Autodesk Inventor part; units mm, degrees
ref_plane "YZ Plane" through (0, 0, 0) normal (1, 0, 0) x (0, 1, 0)
ref_plane "XZ Plane" through (0, 0, 0) normal (0, 1, 0) x (-1, 0, 0)
ref_plane "XY Plane" through (0, 0, 0) normal (0, 0, 1) x (1, 0, 0)
sketch "スケッチ1" plane through (0, 0, 0) normal (0, 0, 1) x (1, 0, 0)
  line L0 (-157.5, 1000) -> (-142.5, 1000)
  line L1 (-142.5, 1000) -> (-142.5, 0)
  line L2 (-142.5, 0) -> (-157.5, 0)
  line L3 (-157.5, 0) -> (-157.5, 1000)
  line L4 (142.5, 500) -> (157.5, 500) construction
  line L5 (157.5, 500) -> (157.5, 0) construction
  line L6 (157.5, 0) -> (142.5, 0)
  line L7 (142.5, 0) -> (142.5, 500) construction
  circle A0 centre (-150, 0) radius 1.6
  circle A1 centre (150, 500) radius 1.6
  line L8 (127.3377, 476.8069) -> (140.2001, 469.0894) construction
  line L9 (140.2001, 469.0894) -> (-127.3377, 23.1931) construction
  line L10 (-127.3377, 23.1931) -> (-140.2001, 30.9106)
  line L11 (-140.2001, 30.9106) -> (127.3377, 476.8069) construction
  line L12 (-150, 0) -> (-133.7689, 27.0518) construction
  circle A2 centre (-150, 1000) radius 1.6
  circle A3 centre (150, 490) radius 1.6
  line L13 (133.7689, 472.9482) -> (150, 500) construction
  line L14 (-133.7689, 27.0518) -> (133.7689, 472.9482) construction
  circle A4 centre (128.6239, 464.3732) radius 1.6
  circle A5 centre (123.479, 455.7983) radius 1.6
  circle A6 centre (118.334, 447.2234) radius 1.6
  circle A7 centre (150, 510) radius 1.6
  circle A8 centre (128.6239, 535.6268) radius 1.6
  circle A9 centre (123.479, 544.2017) radius 1.6
  circle A10 centre (118.334, 552.7766) radius 1.6
  line L15 (157.5, 517.5) -> (157.5, 482.5)
  line L16 (157.5, 482.5) -> (148.2464, 482.5)
  line L17 (157.5, 517.5) -> (148.2464, 517.5)
  line L18 (148.2464, 517.5) -> (120.9065, 563.0665)
  line L19 (120.9065, 563.0665) -> (108.0441, 555.3491)
  line L20 (108.0441, 555.3491) -> (136.6231, 507.7174)
  line L21 (148.2464, 482.5) -> (120.9065, 436.9335)
  line L22 (120.9065, 436.9335) -> (108.0441, 444.6509)
  line L23 (108.0441, 444.6509) -> (136.6231, 492.2826)
  arc A11 (136.6231, 492.2826) -> (136.6231, 507.7174) centre (123.7607, 500) ccw
  line L24 (118.334, 552.7766) -> (128.6239, 535.6268) construction
  point P0 (0, 0)
  point P1 (150, 0)
  dimension "d0" = 15
  dimension "d1" = 15
  dimension "d2" = 1000
  dimension "d3" = 500
  dimension "d4" = 3.2
  dimension "d5" = 3.2
  dimension "d6" = 285
  dimension "d7" = 142.5
  dimension "d8" = 15
  dimension "d9" = 7.5
  dimension "d10" = 520
  dimension "d11" = 3.2
  dimension "d12" = 3.2
  dimension "d13" = 10
  dimension "d14" = 3.2
  dimension "d15" = 3.2
  dimension "d16" = 3.2
  dimension "d17" = 10
  dimension "d18" = 10
  dimension "d19" = 10
  dimension "d20" = 3.2
  dimension "d21" = 10
  dimension "d22" = 7.5
  dimension "d23" = 7.5
  dimension "d24" = 7.5
  dimension "d25" = 7.5
  dimension "d26" = 7.5
  dimension "d27" = 7.5
  dimension "d28" = 7.5
  dimension "d30" = 7.5
  dimension "d31" = 7.5
  dimension "d32" = 15
extrude "押し出し1" add sketch "スケッチ1" along normal blind 3 contours L15 L16 L21 L22 L23 A11 L20 L19 L18 L17
fillet "フィレット1" radius 2 8 edges at (120.9065, 563.0665, 1.5) (157.5, 517.5, 1.5) (157.5, 482.5, 1.5) (120.9065, 436.9335, 1.5) (108.0441, 444.6509, 1.5) (148.2464, 482.5, 1.5) (148.2464, 517.5, 1.5) (108.0441, 555.3491, 1.5)
properties part number "プレート保持_固定具2" material "アルミニウム 6061"
Part model, mm, in its own coordinate system. A direction names the side the tool comes from. Round coordinates to 2 decimals unless told otherwise and drop trailing zeros. Order: outer loops, then holes, each group sorted by start corner. A loop starts at its lowest first (then second) coordinate and runs counter-clockwise, first axis right, second up. Notation, with made-up numbers: M 88,-14.5 L 105,-14.5 A24 ccw 105,21.5 Z; hole C 40.25,-36.75 d9. An arc over 180 degrees is marked long. Put each result on its own line as item: value. Start each with the question number.
1. Drill centre lines: probe 1 along Y at (x, z) = (150, 1.1); probe 2 along Y at (x, z) = (119, 2.7); probe 3 along X at (y, z) = (500, 0.75). Where is each one in solid material? Low to high. Write a range as [from, to].
2. Slice it at A-A on y = 500. List the corners of the cut face in (x, z).
3. Slice it at B-B on z = 2.1. State how many separate pieces and enclosed holes the cut face has, then the cut area to 3 significant figures.
4. Two-plate mould, pull along X, no slides. Class faces 4 (the face through (122.655, 530.997, 1.479)), 5 (the face through (120.68, 437.73, 1.52)), 6 (the face through (128.416, 462.787, 1.479)): +X half, -X half, draft (parallel to the pull), parting line (faces both ways), or undercut.
5. Slice it at C-C on x = 114.5. List the corners of the cut face in (y, z).
6. Tool access for faces 1 (the face through (114.541, 440.753, 1.479)), 2 (the face through (152, 482.5, 1)), 3 (the face through (122.655, 469.003, 1.479)): list every direction of +Z, -Z, +X, -X, +Y, -Y with a clear straight run to the whole face (end or side of a thin tool).
7. Drop a flat-ended pin along its axis: pin 1 (1.5 mm diameter, centred on y = 534.5, z = 2.5, fed in from -X). Give the stop position or say it passes through.
8. Slice it at D-D on y = 471. List the corners of the cut face in (x, z).
Findings:
1. probe 1: [482.5, 488.4], [491.6, 498.4], [501.6, 508.4], [511.6, 517.5]
1. probe 2: [438.08, 445.77], [448.68, 462.91], [537.09, 551.32], [554.23, 561.92]
1. probe 3: [138.76, 148.4], [151.6, 157.5]
2. outline: M 138.76,0 L 148.4,0 L 148.4,3 L 138.76,3 Z; M 151.6,0 L 157.5,0 L 157.5,3 L 151.6,3 Z
3. separate pieces: 1
3. enclosed holes: 9
3. area: 2,150 mm2
4. face 4: -X half
4. face 5: parting line
4. face 6: undercut
5. outline: M 440.78,0 L 455.41,0 L 455.41,3 L 440.78,3 Z; M 544.59,0 L 559.22,0 L 559.22,3 L 544.59,3 Z
6. face 1: +Z, -Z, -X, -Y
6. face 2: +Z, -Z, +X, -Y
6. face 3: +Z, -Z, -X
7. pin 1: x = 120.1
8. outline: M 123.85,0 L 141.35,0 L 141.35,3 L 123.85,3 Z
